from build123d import *

# Parameters (mm, degrees)
F0_R     = 38.25
F1_DEPTH = 0.9
F2_R     = 38.25
F2_R_2   = 37.45
F3_DEPTH = 3
F4_R     = 2.5
F5_R     = 0.7


with BuildPart() as f1:
    # F0 (on Top) → F1 (new body)
    with BuildSketch(Plane.XY):
        Circle(F0_R)
        with BuildLine():
            ThreePointArc((2.4, 3.1372758884), (3.5413627321, 1.7496428207), (3.95, 0))
            ThreePointArc((3.95, 0), (3.5413627321, -1.7496428207), (2.4, -3.1372758884))
            ThreePointArc((2.4, -3.1372758884), (0, -3.95), (-2.4, -3.1372758884))
            ThreePointArc((-2.4, -3.1372758884), (-3.95, 0), (-2.4, 3.1372758884))
            ThreePointArc((-2.4, 3.1372758884), (0, 3.95), (2.4, 3.1372758884))
        make_face(mode=Mode.SUBTRACT)
        with BuildLine():
            Line((-2.4, -3.1372758884), (-2.4, 3.1372758884))
            ThreePointArc((-2.4, 3.1372758884), (-3.95, 0), (-2.4, -3.1372758884))
        make_face()
    extrude(amount=F1_DEPTH)

    # F2 (on face) → F3 (join)
    with BuildSketch(Plane.XY.offset(0.9)):
        Circle(F2_R)
        Circle(F2_R_2, mode=Mode.SUBTRACT)
        with BuildLine():
            Line((-3.2, 3.5103418637), (-3.2, -3.5103418637))
            ThreePointArc((-3.2, -3.5103418637), (4.75, 0), (-3.2, 3.5103418637))
        make_face()
        with BuildLine():
            ThreePointArc((-2.4, 3.1372758884), (3.95, 0), (-2.4, -3.1372758884))
            Line((-2.4, -3.1372758884), (-2.4, 3.1372758884))
        make_face(mode=Mode.SUBTRACT)
    extrude(amount=F3_DEPTH)

    # F4
    f4_edges = [f1.edges().sort_by_distance(p)[0] for p in [
        (-37.45, 0, 0.9),
        (-3.2, 0, 0.9),
        (4.75, 0, 0.9),
    ]]
    fillet(f4_edges, radius=F4_R)

    # F5
    f5_edges = [f1.edges().sort_by_distance(p)[0] for p in [
        (-38.25, 0, 0),
    ]]
    fillet(f5_edges, radius=F5_R)


solid = f1.part
Verification items for the finished model (mm, model axes). A direction names the side the tool comes from. Coordinates: 2 decimals unless noted, no trailing zeros. Order: outer loops, then holes, each group sorted by start corner. A loop starts at its lowest first (then second) coordinate and runs counter-clockwise, first axis right, second up. Notation, with made-up numbers: M 61.5,78 L 106.5,78 A31 cw 106.5,112 Z; hole C -17,47.25 d2. An arc over 180 degrees is marked long. One line per item, written item: value. Start each with the question number.
Item 1: Gauge pin test, flat ends, axial feed: pin 1 (1.5 mm diameter, centred on y = -27.5, z = 1.5, fed in from +X); pin 2 (1 mm diameter, centred on x = 11.5, z = 1, fed in from +Y); pin 3 (1.5 mm diameter, centred on x = 15.5, y = -6.5, fed in from +Z). Record the tip position at first contact, or that the pin passes through.
Item 2: Mould release check, pull along Y, two halves, no side actions. Record for faces 1 (the cylindrical face through (-3.952, -0.063, 1.613)), 2 (the flat face through (-3, 0, 3.9)), 3 (the cylindrical face through (-30.354, -23.275, 2.278)): released by +Y, released by -Y, zero draft, split by the parting line, or undercut.
Item 3: Sectioned sample at A-A (z = 2.2). Enter the section's corners in (x, y).
Item 4: Scan lines: probe 1 along Y at (x, z) = (0, 3.65); probe 2 along Z at (x, y) = (17, -19.5); probe 3 along Y at (x, z) = (-18, 1.8). Record each from-to range of solid material in increasing order.
Item 5: Access from +Z, -Z, +X, -X, +Y, -Y to the whole of each face (thin tool, end or side, straight path). Record for faces 4 (the flat face through (-2.4, 0, 2)), 5 (the flat face through (28.2, -25.3, 3.9)), 6 (the flat face through (0, 8, 0.9)).
Conclusion:
1. pin 1: stops at x = 27.34
1. pin 2: stops at y = 36.63
1. pin 3: stops at z = 0.9
2. face 1: undercut
2. face 2: zero draft
2. face 3: split by the parting line
3. outline: C 0,0 d76.5; M -3.51,-3.64 A5.06 ccw long -3.51,3.64 Z; hole C 0,0 d74.29; hole M -2.4,-3.14 A3.95 ccw long -2.4,3.14 Z
4. probe 1: y = -38.25 to -37.45, -4.75 to -3.95, 3.95 to 4.75, 37.45 to 38.25
4. probe 2: z = 0 to 0.9
4. probe 3: y = -33.75 to -32.18, 32.18 to 33.75
5. face 4: +Z, -Z
5. face 5: +Z, +X, -X, +Y, -Y
5. face 6: +Z
